from build123d import *

# Parameters (mm, degrees)
F0_W     = 8
F0_H     = 3
F1_DEPTH = 10


with BuildPart() as f1:
    # F0 (on Top) → F1 (new body)
    with BuildSketch(Plane.XY):
        with BuildLine():
            Line((-2.316006, 0), (-24, 0))
            Line((-24, 0), (-24, -4))
            Line((-24, -4), (0, -4))
            ThreePointArc((0, -4), (-1.328315, -2.098611), (-2.316006, 0))
        make_face()
        with BuildLine():
            Line((-24, 13.5), (-24, 9.5))
            Line((-24, 9.5), (-16, 9.5))
            Line((-16, 9.5), (-2.316006, 9.5))
            ThreePointArc((-2.316006, 9.5), (-1.328315, 11.598611), (0, 13.5))
            Line((0, 13.5), (-24, 13.5))
        make_face()
        with Locations((-20, 8)):
            Rectangle(F0_W, F0_H)
        with BuildLine():
            ThreePointArc((0, 13.5), (-1.328315, 11.598611), (-2.316006, 9.5))
            Line((-2.316006, 9.5), (0, 9.5))
            Line((0, 9.5), (0, 13.5))
        make_face()
        with BuildLine():
            ThreePointArc((24.167937, 4.75), (15.152911, 17.601573), (0, 13.5))
            Line((0, 13.5), (0, 9.5))
            Line((0, 9.5), (1.13584, 9.5))
            ThreePointArc((1.13584, 9.5), (12.941958, 14.962093), (21, 4.75))
            ThreePointArc((21, 4.75), (12.941958, -5.462093), (1.13584, 0))
            Line((1.13584, 0), (0, 0))
            Line((0, 0), (0, -4))
            ThreePointArc((0, -4), (15.152911, -8.101573), (24.167937, 4.75))
        make_face()
        with BuildLine():
            Line((0, 0), (-2.316006, 0))
            ThreePointArc((-2.316006, 0), (-1.328315, -2.098611), (0, -4))
            Line((0, -4), (0, 0))
        make_face()
    extrude(amount=F1_DEPTH)


solid = f1.part
Read the model definition and answer for the solid it produces. Units are mm, in the model's axes. A direction names the side the tool comes from. Round coordinates to 2 decimals unless told otherwise and drop trailing zeros. Loops run counter-clockwise (first coordinate to the right, second up) from the corner with the lowest first, then second, coordinate; pieces in that order, holes last.
Q1. Each of these flat-tipped pins is pushed along its axis until it touches: pin 1 (0.9 mm diameter, centred on y = 7.5, z = 7, fed in from +X); pin 2 (6 mm diameter, centred on x = 4.5, z = 5.5, fed in from +Y); pin 3 (5 mm diameter, centred on x = -9, z = 5.5, fed in from +Y). Where does it stop, or does it pass through?
Q2. Section C-C on y = 14.75 is taken. Write down the section's boundary in (x, z).
Q3. Section A-A on x = -10 is taken. Write down the section's boundary in (y, z).
Q4. Consider probe 1 along Y at (x, z) = (-5, 7); probe 2 along Y at (x, z) = (10.5, 4.75); probe 3 along X at (y, z) = (11.5, 1). Determine where each line is inside the solid, lowest interval first.
Q5. Determine the mould class of faces 1 (the face through (-8, 9.5, 5)), 2 (the face through (-12, -4, 5)), 3 (the face through (-12, 13.5, 5)), 4 (the face through (0, 10, 10)) for opening direction Y: released by +Y, released by -Y, zero draft, split by the parting line, or undercut.
Q6. Section D-D on y = -6.5 is taken. Write down the section's boundary in (x, z), and give its area (3 significant figures).
Q7. Which of the six approach directions +Z, -Z, +X, -X, +Y, -Y give full straight-line access (tool end or side, diameter ignored) to faces 5 (the face through (-11, 0, 5)), 6 (the face through (-16, 8, 5)), 7 (the face through (-24, 10, 5))?
Q8. Section B-B on z = 1 is taken. Write down the section's boundary in (x, y), and give its area (3 significant figures).
Output:
1. pin 1: stops at x = 23.97
1. pin 2: stops at y = 18.08
1. pin 3: stops at y = 13.5
2. outline: (1.18, 0) - (7.3, 0) - (7.3, 10) - (1.18, 10) - close; (13.7, 0) - (19.82, 0) - (19.82, 10) - (13.7, 10) - close
3. outline: (-4, 0) - (0, 0) - (0, 10) - (-4, 10) - close; (9.5, 0) - (13.5, 0) - (13.5, 10) - (9.5, 10) - close
4. probe 1: y = -4 to 0, 9.5 to 13.5
4. probe 2: y = -8.92 to -5.75, 15.25 to 18.42
4. probe 3: x = -24 to 2.46, 18.54 to 22.38
5. face 1: undercut
5. face 2: released by -Y
5. face 3: released by +Y
5. face 4: zero draft
6. outline: (2.74, 0) - (18.26, 0) - (18.26, 10) - (2.74, 10) - close
6. area: 155 mm2
7. face 5: +Z, -Z, -X
7. face 6: +Z, -Z
7. face 7: +Z, -Z, -X, +Y, -Y
8. outline: (-24, -4) - (0, -4) arc R13.67 ccw (long way) to (0, 13.5) - (-24, 13.5) - (-24, 6.5) - (-16, 6.5) - (-16, 9.5) - (1.14, 9.5) arc R10.5 cw (long way) to (1.14, 0) - (-24, 0) - close
8. area: 415 mm2
